```python
from build123d import *

# Parameters (mm, degrees)
F0_W          = 25.4
F0_H          = 19.05
F1_DEPTH      = 19.05
F2_DEPTH      = 6.35
F4_DEPTH      = 3.175
F4_DEPTH_BACK = 25.4
F5_R          = 11.8364
F6_DEPTH      = 50.8
F7_R          = 3.81
F8_DEPTH      = 25.4


with BuildPart() as f1:
    # F0 (on Front) → F1 (new body, symmetric)
    with BuildSketch(Plane.XZ):
        with BuildLine():
            Line((22.225, 9.525), (41.275, 9.525))
            Line((41.275, 9.525), (41.275, 27.3961414351))
            ThreePointArc((41.275, 27.3961414351), (44.7413406712, 37.2976968008), (53.6265966817, 42.8752))
            Line((53.6265966817, 42.8752), (60.325, 42.8752))
            Line((60.325, 42.8752), (60.325, 61.9252))
            Line((60.325, 61.9252), (51.9059805855, 61.9252))
            ThreePointArc((51.9059805855, 61.9252), (30.6650702941, 50.1624350173), (22.225, 27.3961414351))
            Line((22.225, 27.3961414351), (22.225, 9.525))
        make_face()
        Polygon((-41.275, -9.525), (41.275, -9.525), (41.275, 9.525), (22.225, 9.525), (-41.275, 9.525), align=None)
        with Locations((73.025, 52.4002)):
            Rectangle(F0_W, F0_H)
    extrude(amount=F1_DEPTH, both=True)

    # F0 (on Front) → F2 (join, symmetric)
    with BuildSketch(Plane.XZ):
        with BuildLine():
            add(Edge.make_bspline(
                [(-41.275, 9.525), (-35.163089633, 38.4709127247), (-8.6453789845, 60.5748556554), (51.9059805855, 61.9252)],
                knots=[0, 0, 0, 0, 106.9040509191, 106.9040509191, 106.9040509191, 106.9040509191], degree=3))
            Line((-41.275, 9.525), (22.225, 9.525))
            Line((22.225, 9.525), (22.225, 27.3961414351))
            ThreePointArc((22.225, 27.3961414351), (30.6650702941, 50.1624350173), (51.9059805855, 61.9252))
        make_face()
    extrude(amount=F2_DEPTH, both=True)

    # F3 (on face) → F4 (join, two sides)
    with BuildSketch(Plane.XY.offset(61.9252)) as f4_sk:
        with BuildLine():
            Line((85.725, -19.05), (85.725, 19.05))
            ThreePointArc((85.725, 19.05), (66.675, 0), (85.725, -19.05))
        make_face()
        with BuildLine():
            ThreePointArc((85.725, -19.05), (99.1953841816, -13.4703841816), (104.775, 0))
            ThreePointArc((104.775, 0), (99.1953841816, 13.4703841816), (85.725, 19.05))
            Line((85.725, 19.05), (85.725, -19.05))
        make_face()
    extrude(amount=F4_DEPTH)
    extrude(f4_sk.sketch, amount=-F4_DEPTH_BACK)

    # F5 (on face) → F6 (cut)
    with BuildSketch(Plane.XY.offset(65.1002)):
        with Locations((85.725, 0)):
            Circle(F5_R)
    extrude(amount=-F6_DEPTH, mode=Mode.SUBTRACT)

    # F7 (on face) → F8 (cut)
    with BuildSketch(Plane.XY.offset(9.525)):
        with Locations((-6.4540371954, -12.6517117023)):
            Circle(F7_R)
        with Locations((-19.1540371954, -12.6517117023)):
            Circle(F7_R)
        with Locations((-31.8540371954, -12.6517117023)):
            Circle(F7_R)
        with Locations((-6.4540371954, 12.6517117023)):
            Circle(F7_R)
        with Locations((-19.1540371954, 12.6517117023)):
            Circle(F7_R)
        with Locations((-31.8540371954, 12.6517117023)):
            Circle(F7_R)
    extrude(amount=-F8_DEPTH, mode=Mode.SUBTRACT)


solid = f1.part
```
For this review, take the finished solid that the model builds, in its own axes (mm). A direction names the side the tool comes from. Round coordinates to 2 decimals unless told otherwise and drop trailing zeros. Loops run counter-clockwise (first coordinate to the right, second up) from the corner with the lowest first, then second, coordinate; pieces in that order, holes last.
Q1. Mouldability with a two-part tool opening along Y and no side actions: class faces 4 (the face through (30.89, 12.61, 50.42)), 5 (the face through (-4, 6.35, 30)), 6 (the face through (-15.52, -11.51, 0.13)) as +Y half, -Y half, draft (parallel to the pull), parting line (faces both ways), or undercut.
Result sheet:
face 4: draft
face 5: +Y half
face 6: undercut
Q2. Insertion check: pin 1 Ø10 at (x, y) = (61, 9.5) entering from +Z; pin 2 Ø8 at (y, z) = (12, 24.5) entering from +X; pin 3 Ø14 at (x, y) = (85.725, 0) entering from -Z; pin 4 Ø19 at (x, y) = (89.5, -7.5) entering from -Z. Each pin has a flat end and moves straight along its axis. Give the tip position at first contact, or say it passes through.
Result sheet:
pin 1: stops at z = 61.93
pin 2: stops at x = 41.31
pin 3: passes through
pin 4: stops at z = 36.53
Q3. Add section B-B on z = 5.5. Write out the cut boundary in (x, y) (3 decimals), plus the area to 3 significant figures.
Result sheet:
outline: (-41.275, -19.05) - (41.275, -19.05) - (41.275, 19.05) - (-41.275, 19.05) - close; hole circle Ø7.62 at (-31.854, -12.652); hole circle Ø7.62 at (-31.854, 12.652); hole circle Ø7.62 at (-19.154, -12.652); hole circle Ø7.62 at (-19.154, 12.652); hole circle Ø7.62 at (-6.454, -12.652); hole circle Ø7.62 at (-6.454, 12.652)
area: 2,870 mm2
Q4. Add section A-A on y = 14. Give the number of separate pieces and of enclosed holes in the cut face, plus the area to 3 significant figures.
Result sheet:
separate pieces: 4
enclosed holes: 0
area: 3,300 mm2
Q5. To check wall thickness, follow line 1 along X through (y, z) = (13, 8) (3 decimals); line 2 along Y through (x, z) = (86, 60); line 3 along Y through (x, z) = (-21.5, -0.5). State the ranges of each line that lie inside material, in increasing order.
Result sheet:
line 1: x = -41.275 to -35.648, -28.06 to -22.948, -15.36 to -10.248, -2.66 to 41.275
line 2: y = -19.05 to -11.83, 11.83 to 19.05
line 3: y = -19.05 to -15.65, -9.65 to 9.65, 15.65 to 19.05
Q6. Machinability: for faces 1 (the face through (-4, -6.35, 30)), 2 (the face through (94, 9, 36.525)), 3 (the face through (44.65, -0.27, 37.18)), which of the approach directions +Z, -Z, +X, -X, +Y, -Y give a long, thin tool a straight path to every point of the face, cutting with its end or side? Answer none if there is none.
Result sheet:
face 1: +Z, -X, -Y
face 2: -Z, +X, +Y, -Y
face 3: -Z, +Y, -Y
